The listing builds one solid part. Answer for the finished solid, in the listing's coordinates (mm). A direction names the side the tool comes from. Coordinates: 2 decimals unless noted, no trailing zeros. Order: outer loops, then holes, each group sorted by start corner. A loop starts at its lowest first (then second) coordinate and runs counter-clockwise, first axis right, second up.
```python
from build123d import *

# Parameters (mm, degrees)
SKETCH1_W                  = 55
SKETCH1_H                  = 65
BASE_DEPTH                 = 2
SKETCH2_R                  = 1.2
PIMOUNTSCREWHOLES_DEPTH    = 2
SKETCH3_W                  = 20
SKETCH3_H                  = 2
PLATELEGEXT_1_DEPTH        = 10
SKETCH19_W                 = 55
SKETCH19_H                 = 2
PIFRONTBASE_DEPTH          = 20
SKETCH21_W                 = 65
SKETCH21_H                 = 2
BATTERYWALL_EXT_DEPTH      = 10
SKETCH22_W                 = 22.5
SKETCH22_H                 = 2
SKETCH22_W_2               = 12.5
PLATELEGEXT_2_DEPTH        = 10
SKETCH30_W                 = 10
SKETCH30_H                 = 2
CORNEREXTENSION_DEPTH      = 10
SKETCH23_W                 = 22.5
SKETCH23_H                 = 5
SKETCH23_W_2               = 5
SKETCH23_H_2               = 20
PLATELEGS_DEPTH            = 50.8
SKETCH29_R                 = 1.5
BATTERY_SCREWHOLES_DEPTH   = 5
ROTATORPLATE_DEPTH         = 10
SKETCH25_W                 = 20
SKETCH25_H                 = 41
INSET_SERVO_DEPTH          = 4
SKETCH26_R                 = 1.5
HOLE_SERVOSCREW_DEPTH      = 6
SKETCH27_R                 = 7
INSET_SERVOAXLE_DEPTH      = 5.8
RETAININGWALLS_SERVO_DEPTH = 10
SKETCH31_W                 = 15
SKETCH31_H                 = 11
POWER_HOLE_DEPTH           = 5


with BuildPart() as part:
    # Sketch1 → Base (new body)
    with BuildSketch(Plane(origin=(0, 0, 0), x_dir=(1, 0, 0), z_dir=(0, 1, 0))):
        with Locations((27.5, 32.5)):
            Rectangle(SKETCH1_W, SKETCH1_H)
    extrude(amount=BASE_DEPTH)

    # Sketch2 → PiMountScrewHoles (cut)
    with BuildSketch(Plane(origin=(0, 2, 0), x_dir=(1, 0, 0), z_dir=(0, 1, 0))):
        with Locations(Location((3, 3.5, 0), (0, 0, 270))):
            Circle(SKETCH2_R)
        with Locations(Location((52, 3.5, 0), (0, 0, 270))):
            Circle(SKETCH2_R)
        with Locations(Location((3, 61.5, 0), (0, 0, 270))):
            Circle(SKETCH2_R)
        with Locations(Location((52, 61.5, 0), (0, 0, 270))):
            Circle(SKETCH2_R)
    extrude(amount=-PIMOUNTSCREWHOLES_DEPTH, mode=Mode.SUBTRACT)

    # Sketch3 → PlateLegExt-1 (add)
    with BuildSketch(Plane.ZY):
        with Locations((-55, 1)):
            Rectangle(SKETCH3_W, SKETCH3_H)
    extrude(amount=PLATELEGEXT_1_DEPTH)

    # Sketch19 → PiFrontBase (add)
    with BuildSketch(Plane(origin=(0, 0, -65), x_dir=(-1, 0, 0), z_dir=(0, 0, -1))):
        with Locations((-27.5, 1)):
            Rectangle(SKETCH19_W, SKETCH19_H)
    extrude(amount=PIFRONTBASE_DEPTH)

    # Sketch21 → BatteryWall-Ext (add)
    with BuildSketch(Plane(origin=(55, 0, 0), x_dir=(0, 0, -1), z_dir=(1, 0, 0))):
        with Locations((32.5, 1)):
            Rectangle(SKETCH21_W, SKETCH21_H)
    extrude(amount=BATTERYWALL_EXT_DEPTH)

    # Sketch22 → PlateLegExt-2 (add)
    with BuildSketch(Plane.XY):
        with Locations((11.25, 1)):
            Rectangle(SKETCH22_W, SKETCH22_H)
        with Locations((48.75, 1)):
            Rectangle(SKETCH22_W_2, SKETCH22_H)
    extrude(amount=PLATELEGEXT_2_DEPTH)

    # Sketch30 → CornerExtension (add)
    with BuildSketch(Plane(origin=(55, 0, 0), x_dir=(0, 0, -1), z_dir=(1, 0, 0))):
        with Locations((-5, 1)):
            Rectangle(SKETCH30_W, SKETCH30_H)
    extrude(amount=CORNEREXTENSION_DEPTH)

    # Sketch23 → PlateLegs (add)
    with BuildSketch(Plane(origin=(0, 2, 0), x_dir=(1, 0, 0), z_dir=(0, 1, 0))):
        with Locations((11.25, -7.5)):
            Rectangle(SKETCH23_W, SKETCH23_H)
        with Locations((-7.5, 55)):
            Rectangle(SKETCH23_W_2, SKETCH23_H_2)
        Polygon((60, 65), (65, 65), (65, -10), (42.5, -10), (42.5, -5), (60, -5), align=None)
    extrude(amount=PLATELEGS_DEPTH)

    # Sketch29 → Battery-ScrewHoles (cut)
    with BuildSketch(Plane(origin=(65, 0, 0), x_dir=(0, 0, -1), z_dir=(1, 0, 0))):
        with Locations((59.045, 35)):
            Circle(SKETCH29_R)
        with Locations((-0.905, 35)):
            Circle(SKETCH29_R)
    extrude(amount=-BATTERY_SCREWHOLES_DEPTH, mode=Mode.SUBTRACT)

    # Sketch24 → RotatorPlate (add)
    with BuildSketch(Plane(origin=(0, 52.8, 0), x_dir=(1, 0, 0), z_dir=(0, 1, 0))):
        Polygon((0, -10), (65, -10), (65, 65), (-10, 65), (-10, 45), align=None)
    extrude(amount=ROTATORPLATE_DEPTH)

    # Sketch25 → Inset-Servo (cut)
    with BuildSketch(Plane(origin=(0, 62.8, 0), x_dir=(1, 0, 0), z_dir=(0, 1, 0))):
        with Locations((27.5, 27.5)):
            Rectangle(SKETCH25_W, SKETCH25_H)
    extrude(amount=-INSET_SERVO_DEPTH, mode=Mode.SUBTRACT)

    # Sketch26 → Hole-ServoScrew (cut)
    with BuildSketch(Plane(origin=(0, 58.8, 0), x_dir=(1, 0, 0), z_dir=(0, 1, 0))):
        with Locations(Location((27.5, 37.75, 0), (0, 0, 270))):
            Circle(SKETCH26_R)
    extrude(amount=-HOLE_SERVOSCREW_DEPTH, mode=Mode.SUBTRACT)

    # Sketch27 → Inset-ServoAxle (cut)
    with BuildSketch(Plane(origin=(0, 58.8, 0), x_dir=(1, 0, 0), z_dir=(0, 1, 0))):
        with Locations(Location((27.5, 37.75, 0), (0, 0, 270))):
            Circle(SKETCH27_R)
    extrude(amount=-INSET_SERVOAXLE_DEPTH, mode=Mode.SUBTRACT)

    # Sketch28 → RetainingWalls-Servo (add)
    with BuildSketch(Plane(origin=(0, 62.8, 0), x_dir=(1, 0, 0), z_dir=(0, 1, 0))):
        Polygon((37.5, 48), (33.5, 48), (33.5, 50), (40, 50), (40, 5), (15, 5), (15, 50), (21.5, 50), (21.5, 48), (17.5, 48), (17.5, 7), (37.5, 7), align=None)
    extrude(amount=RETAININGWALLS_SERVO_DEPTH)

    # Sketch31 → Power-Hole (cut)
    with BuildSketch(Plane.ZY.offset(-60)):
        with Locations((-15.5, 7.5)):
            Rectangle(SKETCH31_W, SKETCH31_H)
    extrude(amount=-POWER_HOLE_DEPTH, mode=Mode.SUBTRACT)


solid = part.part
```
1) A cutting plane is placed at C-C, the plane z = -54.5. Write down the section's boundary in (x, y), plus the area to 3 significant figures.
2) Each of these flat-tipped pins is pushed along its axis until it touches: P1, Ø12, axis at x = 55, y = 28.5, coming from the -Z side; P2, Ø10, axis at y = 59.5, z = -24.5, coming from the -X side; P3, Ø3, axis at x = 3, z = -3.5, coming from the +Y side. Where does it stop, or does it pass through?
3) A cutting plane is placed at B-B, the plane y = 4.5. Write down the section's boundary in (x, z).
4) For faces 1 (the flat face through (51, 27, 5)), 2 (the cylindrical face through (62.535, 34.425, -60.431)), 3 (the cylindrical face through (4.01, 1.01, -2.85)), 4 (the flat face through (37.5, 66, -27)), determine the directions among +Z, -Z, +X, -X, +Y, -Y from which every point of the face is accessible in a straight line to the end or side of a thin tool.
5) A cutting plane is placed at D-D, the plane y = 46. Write down the section's boundary in (x, z).
6) Straight lines are drawn through the part: probe 1 along X at (y, z) = (1, -61.5); probe 2 along Y at (x, z) = (50, -12); probe 3 along X at (y, z) = (1.3, -3.5). For each, find the intervals that lie inside material, in ascending order.
7) The mould has two halves that part along Y. Classify faces 5 (the flat face through (25, 55, -65)), 6 (the flat face through (62, 7, -23)), 7 (the flat face through (17, 72.8, -24)): released by +Y, released by -Y, zero draft, split by the parting line, or undercut.
8) A cutting plane is placed at A-A, the plane x = -3. Write down the section's boundary in (y, z).
Working result:
1. outline: (-10, 0) - (65, 0) - (65, 62.8) - (-10, 62.8) - close; hole (-5, 2) - (60, 2) - (60, 52.8) - (-5, 52.8) - close
1. area: 1,410 mm2
2. P1: stops at z = -65
2. P2: stops at x = -7.18
2. P3: stops at y = 62.8
3. outline: (-10, -65) - (-5, -65) - (-5, -45) - (-10, -45) - close; (0, 5) - (22.5, 5) - (22.5, 10) - (0, 10) - close; (42.5, 5) - (60, 5) - (60, -8) - (65, -8) - (65, 10) - (42.5, 10) - close; (60, -65) - (65, -65) - (65, -23) - (60, -23) - close
4. face 1: -Z, -X
4. face 2: +X
4. face 3: -Y
4. face 4: +Y
5. outline: (-10, -65) - (-5, -65) - (-5, -45) - (-10, -45) - close; (0, 5) - (22.5, 5) - (22.5, 10) - (0, 10) - close; (42.5, 5) - (60, 5) - (60, -65) - (65, -65) - (65, 10) - (42.5, 10) - close
6. probe 1: x = -10 to 1.8, 4.2 to 50.8, 53.2 to 65
6. probe 2: y = 0 to 2, 52.8 to 62.8
6. probe 3: x = 0 to 1.8, 4.2 to 50.8, 53.2 to 65
7. face 5: zero draft
7. face 6: undercut
7. face 7: released by +Y
8. outline: (0, -65) - (2, -65) - (2, -45) - (0, -45) - close; (52.8, -65) - (62.8, -65) - (62.8, -6.5) - (52.8, -6.5) - close
